from build123d import *

# Parameters (mm, degrees)
CROQUIS1_W               = 53.24
CROQUIS1_H               = 35.28
CROQUIS1_W_2             = 46.88
CROQUIS1_H_2             = 29.18
SALIENTE_EXTRUIR2_DEPTH  = 41.2
CROQUIS3_W               = 48.88
CROQUIS3_H               = 33.1
CROQUIS3_W_2             = 40.02
CROQUIS3_H_2             = 25.75
SALIENTE_EXTRUIR11_DEPTH = 50
CROQUIS21_W              = 51.220456713
CROQUIS21_H              = 38.403596391
CORTAR_EXTRUIR1_DEPTH    = 24
CROQUIS22_W              = 52.73
CROQUIS22_H              = 48.22
SALIENTE_EXTRUIR15_DEPTH = 2.92
CROQUIS24_W              = 40.02
CROQUIS24_H              = 25.75
CORTAR_EXTRUIR2_DEPTH    = 81.92


with BuildPart() as part:
    # Croquis1 → Saliente-Extruir2 (new body)
    with BuildSketch(Plane.XY):
        with Locations((-10.511813518, 0.307314635)):
            Rectangle(CROQUIS1_W, CROQUIS1_H)
        with Locations((-10.511813518, 0.437314635)):
            Rectangle(CROQUIS1_W_2, CROQUIS1_H_2, mode=Mode.SUBTRACT)
    extrude(amount=SALIENTE_EXTRUIR2_DEPTH)

    # Croquis3 → Saliente-Extruir11 (add)
    with BuildSketch(Plane.XY.offset(41.2)):
        with Locations((-10.511813518, 1.397314635)):
            Rectangle(CROQUIS3_W, CROQUIS3_H)
        with Locations((-10.511813518, 2.152314635)):
            Rectangle(CROQUIS3_W_2, CROQUIS3_H_2, mode=Mode.SUBTRACT)
    extrude(amount=SALIENTE_EXTRUIR11_DEPTH)

    # Croquis21 → Cortar-Extruir1 (cut)
    with BuildSketch(Plane(origin=(0, 32.232144696, 69.095644301), x_dir=(-1, 0, 0), z_dir=(0, -0.4227509471843472, -0.906245902972663))):
        with Locations((10.82223744, -34.046833933)):
            Rectangle(CROQUIS21_W, CROQUIS21_H)
    extrude(amount=-CORTAR_EXTRUIR1_DEPTH, mode=Mode.SUBTRACT)

    # Croquis22 → Saliente-Extruir15 (add)
    with BuildSketch(Plane(origin=(0, 32.232144696, 69.095644301), x_dir=(-1, 0, 0), z_dir=(0, -0.4227509471843472, -0.906245902972663))):
        with Locations((10.511813518, -39.872642362)):
            Rectangle(CROQUIS22_W, CROQUIS22_H)
    extrude(amount=SALIENTE_EXTRUIR15_DEPTH)

    # Croquis24 → Cortar-Extruir2 (cut)
    with BuildSketch(Plane.XY.offset(41.2)):
        with Locations((-10.511813518, 2.152314635)):
            Rectangle(CROQUIS24_W, CROQUIS24_H)
    extrude(amount=CORTAR_EXTRUIR2_DEPTH, mode=Mode.SUBTRACT)


solid = part.part
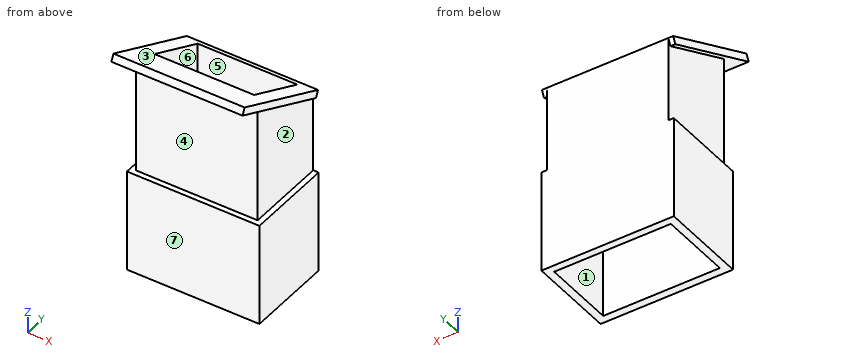
Build history of the part. All positions in model axes, mm. Face numbers are marked on the shaded views. A direction names the side the tool comes from. Round coordinates to 2 decimals unless told otherwise and drop trailing zeros. Write each loop counter-clockwise with the first axis right and the second up, starting at its lowest first coordinate (ties: lowest second). Pieces come first, ordered by that corner, then holes. Notation, with made-up numbers: (54, 14) - (101, 14) arc R11 cw to (101, 22) - close; hole circle Ø10 at (41.25, -9). An arc over 180 degrees is marked (long way). One line per question, with ' | ' between items.
1. Drill centre lines: line 1 along X through (y, z) = (-8, 33); line 2 along X through (y, z) = (-9, 68); line 3 along Y through (x, z) = (-22, 57). Where is each one in solid material? Low to high. Write a range as from..to.
Results are:
line 1: -37.13..-33.95, 12.93..16.11 | line 2: -34.95..-30.52, 9.5..13.93 | line 3: -15.15..-10.72, 15.03..17.95
2. Mould opens along Z. For the marked faces 1, 2 and 3 say: released by +Z, released by -Z, zero draft, split by the parting line, or undercut.
Results are:
face 1: zero draft | face 2: undercut | face 3: released by +Z
3. Tool access for the marked faces 4, 5, 6 and 7: list every direction of +Z, -Z, +X, -X, +Y, -Y with a clear straight run to the whole face (end or side of a thin tool).
Results are:
face 4: +X, -X, -Y | face 5: -Z | face 6: +Z, -Z | face 7: -Z, +X, -X, -Y
4. Band-saw the part on A-A, the plane x = 1. Write the cut outline in (y, z).
Results are:
outline: (-26.99, 93.5) - (-15.15, 87.98) - (-15.15, 41.2) - (-17.33, 41.2) - (-17.33, 0) - (-14.15, 0) - (-14.15, 41.2) - (-10.72, 41.2) - (-10.72, 89.13) - (-25.75, 96.14) - close; (15.03, 0) - (17.95, 0) - (17.95, 75.76) - (15.03, 77.12) - close
5. Band-saw the part on B-B, the plane z = 49.5. Write the cut outline in (x, y), and give its area (3 significant figures).
Results are:
outline: (-34.95, -15.15) - (13.93, -15.15) - (13.93, 17.95) - (-34.95, 17.95) - close; hole (-30.52, -10.72) - (9.5, -10.72) - (9.5, 15.03) - (-30.52, 15.03) - close | area: 587 mm^2
6. Band-saw the part on C-C, the plane y = 12.5. Write the cut outline in (x, z), and give its area (3 significant figures).
Results are:
outline: (-37.13, 0) - (-33.95, 0) - (-33.95, 41.2) - (-30.52, 41.2) - (-30.52, 78.3) - (-36.88, 78.3) - (-36.88, 75.08) - (-34.95, 75.08) - (-34.95, 41.2) - (-37.13, 41.2) - close; (9.5, 41.2) - (12.93, 41.2) - (12.93, 0) - (16.11, 0) - (16.11, 41.2) - (13.93, 41.2) - (13.93, 75.08) - (15.85, 75.08) - (15.85, 78.3) - (9.5, 78.3) - close | area: 603 mm^2
7. Drop flat-ended pins along their axis: pin 1 Ø7.5 at (y, z) = (-0.5, 73.5) entering from -X; pin 2 Ø11.5 at (y, z) = (-5.5, 82.5) entering from +X; pin 3 Ø14 at (x, z) = (-10.5, 58) entering from -Y. Give the stop position or say it passes through.
Results are:
pin 1: x = -34.95 | pin 2: x = 15.85 | pin 3: y = -15.15
8. Band-saw the part on D-D, the plane z = 28. Write the cut outline in (x, y), and give its area (3 significant figures).
Results are:
outline: (-37.13, -17.33) - (16.11, -17.33) - (16.11, 17.95) - (-37.13, 17.95) - close; hole (-33.95, -14.15) - (12.93, -14.15) - (12.93, 15.03) - (-33.95, 15.03) - close | area: 510 mm^2
